```python
from build123d import *

# Parameters (mm, degrees)
F0_W     = 2
F0_H     = 115
F1_DEPTH = 20
F2_DEPTH = 20
F0_W_2   = 80
F0_R     = 15
F3_DEPTH = 2
F0_R_2   = 13
F4_DEPTH = 12
F5_DEPTH = 10
F6_SIZE  = 0.5
F7_SIZE  = 1


with BuildPart() as f1:
    # F0 (on Front) → F1 (new body)
    with BuildSketch(Plane.XZ):
        with Locations((-41, 0)):
            Rectangle(F0_W, F0_H)
    extrude(amount=-F1_DEPTH)



with BuildPart() as f2:
    # F0 (on Front) → F2 (new body)
    with BuildSketch(Plane.XZ):
        with Locations((41, 0)):
            Rectangle(F0_W, F0_H)
    extrude(amount=-F2_DEPTH)


with BuildPart() as f1_1:
    add(f1.part)

    add(f2.part)  # F3 merges F2
    # F0 (on Front) → F3 (join)
    with BuildSketch(Plane.XZ):
        Rectangle(F0_W_2, F0_H)
        Circle(F0_R, mode=Mode.SUBTRACT)
        with Locations((41, 0)):
            Rectangle(F0_W, F0_H)
        with Locations((-41, 0)):
            Rectangle(F0_W, F0_H)
    extrude(amount=F3_DEPTH)

    # F0 (on Front) → F4 (join)
    with BuildSketch(Plane.XZ):
        Circle(F0_R)
        Circle(F0_R_2, mode=Mode.SUBTRACT)
        Circle(F0_R_2)
    extrude(amount=F4_DEPTH)

    # F0 (on Front) → F5 (cut)
    with BuildSketch(Plane.XZ):
        Circle(F0_R_2)
    extrude(amount=F5_DEPTH, mode=Mode.SUBTRACT)

    # F6
    f6_edges = [f1_1.edges().sort_by_distance(p)[0] for p in [
        (42, -2, 0),
        (0, -2, 57.5),
        (-42, -2, 0),
        (0, -2, -57.5),
        (-15, -2, 0),
    ]]
    chamfer(f6_edges, length=F6_SIZE)

    # F7
    f7_edges = [f1_1.edges().sort_by_distance(p)[0] for p in [
        (-15, -12, 0),
    ]]
    chamfer(f7_edges, length=F7_SIZE)


solid = f1_1.part
```
Verification items for the finished model (mm, model axes). A direction names the side the tool comes from. Give positions to 0.01 mm unless a question says otherwise; leave off trailing zeros. Order: outer loops, then holes, each group sorted by start corner. A loop starts at its lowest first (then second) coordinate and runs counter-clockwise, first axis right, second up. Notation, with made-up numbers: M 57.5,83 L 113.5,83 A7 cw 113.5,90 Z; hole C 23,4.5 d8. An arc over 180 degrees is marked long. Return JSON: item names as keys, results as strings. Group by question number.
1) Section check C-C on x = 0. Record the cut outline in (y, z), and give its area (3 significant figures).
2) Access from +Z, -Z, +X, -X, +Y, -Y to the whole of each face (thin tool, end or side, straight path). Record for faces 5 (the face through (40, 10, -1)), 6 (the face through (-10.316, -4.93, -7.91)), 7 (the face through (-0.2, -0.3, -57.5)).
3) Go/stop test with flat-tipped pins: pin 1 Ø1.5 at (x, y) = (-32.5, 1) entering from +Z (1 decimal); pin 2 Ø2 at (x, z) = (-33, 39.5) entering from -Y; pin 3 Ø10 at (y, z) = (-8.5, 3) entering from +X; pin 4 Ø8 at (x, z) = (6, -6.5) entering from +Y. Record where each tip stops, or that it passes through.
4) Scan lines: line 1 (Z direction, x = 0, y = -6); line 2 (X direction, y = 4.5, z = -11.5); line 3 (Y direction, x = 1, z = 9). Record each from-to range of solid material in increasing order.
5) Section check A-A on y = 6. Record the cut outline in (x, z), and give its area (3 significant figures).
6) Section check D-D on z = -48. Record the cut outline in (x, y).
7) Section check B-B on z = 0. Record the cut outline in (x, y), and give its area (3 significant figures).
8) Mould release check, pull along X, two halves, no side actions. Record for faces 1 (the face through (0, -10, 0)), 2 (the face through (9, -2, 13)), 3 (the face through (-14.985, -6.69, 0.66)), 4 (the face through (-40, 10, -1)): pulls with the +X half, pulls with the -X half, needs draft (parallel to the pull), parting line crosses it, or undercut.
Answer block:
{
 "1": {"outline": "M -12,-14 L -11,-15 L -2.5,-15 L -2,-15.5 L -2,-57 L -1.5,-57.5 L 0,-57.5 L 0,-13 L -10,-13 L -10,13 L 0,13 L 0,57.5 L -1.5,57.5 L -2,57 L -2,15.5 L -2.5,15 L -11,15 L -12,14 Z", "area": "269 mm^2"},
 "2": {"face 5": "+Z, -Z, +Y", "face 6": "+Y", "face 7": "-Z, +X, -X, +Y, -Y"},
 "3": {"pin 1": "passes through", "pin 2": "stops at y = -2", "pin 3": "stops at x = 15", "pin 4": "stops at y = -10"},
 "4": {"line 1": "z = -15 to -13, 13 to 15", "line 2": "x = -42 to -40, 40 to 42", "line 3": "y = -12 to -10"},
 "5": {"outline": "M -42,-57.5 L -40,-57.5 L -40,57.5 L -42,57.5 Z; M 40,-57.5 L 42,-57.5 L 42,57.5 L 40,57.5 Z", "area": "460 mm^2"},
 "6": {"outline": "M -42,-1.5 L -41.5,-2 L 41.5,-2 L 42,-1.5 L 42,20 L 40,20 L 40,0 L -40,0 L -40,20 L -42,20 Z"},
 "7": {"outline": "M -42,-1.5 L -41.5,-2 L -15.5,-2 L -15,-2.5 L -15,-11 L -14,-12 L 14,-12 L 15,-11 L 15,-2.5 L 15.5,-2 L 41.5,-2 L 42,-1.5 L 42,20 L 40,20 L 40,0 L 13,0 L 13,-10 L -13,-10 L -13,0 L -40,0 L -40,20 L -42,20 Z", "area": "287 mm^2"},
 "8": {"face 1": "undercut", "face 2": "needs draft", "face 3": "parting line crosses it", "face 4": "undercut"}
}
